from build123d import *

# Parameters (mm, degrees)
ESBO_O1_W                          = 90
ESBO_O1_H                          = 93
RESSALTO_EXTRUS_O1_DEPTH           = 12.7
ESBO_O3_R                          = 32.51
CORTE_EXTRUS_O2_DEPTH              = 66.943460631
CORTE_EXTRUS_O4_REACH              = 67.943
ESBO_O5_W                          = 27.5
ESBO_O5_H                          = 13
CORTE_EXTRUS_O5_REACH              = 67.943
ESBO_O6_W                          = 7
ESBO_O6_H                          = 26.329700269
CORTE_EXTRUS_O6_REACH              = 80.929
ESBO_O7_R                          = 2.5
CORTE_EXTRUS_O7_REACH              = 80.929
CORTE_EXTRUS_O8_DEPTH              = 66.943460631
TALADRO_DE_MARGEN_PARA_00001_D     = 5
TALADRO_DE_MARGEN_PARA_00001_DEPTH = 20
TALADRO_DE_MARGEN_PARA_00001_TIP   = 1.502151548


with BuildPart() as part:
    # Esboço1 → Ressalto-extrusão1 (new body)
    with BuildSketch(Plane(origin=(0, 0, 0), x_dir=(1, 0, 0), z_dir=(0, 1, 0))):
        Rectangle(ESBO_O1_W, ESBO_O1_H)
    extrude(amount=RESSALTO_EXTRUS_O1_DEPTH)

    # Esboço3 → Corte-extrusão2 (cut, through all)
    with BuildSketch(Plane(origin=(0, 12.7, 0), x_dir=(1, 0, 0), z_dir=(0, 1, 0))):
        with Locations(Location((0, 3.5, 0), (0, 0, 270))):
            Circle(ESBO_O3_R)
    extrude(amount=-CORTE_EXTRUS_O2_DEPTH, mode=Mode.SUBTRACT)

    # Esboço5 → Corte-extrusão4 (cut, up to next)
    with BuildSketch(Plane(origin=(0, 12.7, 0), x_dir=(1, 0, 0), z_dir=(0, 1, 0)), mode=Mode.PRIVATE) as corte_extrus_o4_sk1:
        with Locations((31.25, -40)):
            Rectangle(ESBO_O5_W, ESBO_O5_H)
    corte_extrus_o4_tool1 = extrude(corte_extrus_o4_sk1.sketch, amount=-CORTE_EXTRUS_O4_REACH, mode=Mode.PRIVATE) & part.part
    # Esboço5 → Corte-extrusão4 (cut, up to next)
    with BuildSketch(Plane(origin=(0, 12.7, 0), x_dir=(1, 0, 0), z_dir=(0, 1, 0)), mode=Mode.PRIVATE) as corte_extrus_o4_sk2:
        with Locations((-31.25, -40)):
            Rectangle(ESBO_O5_W, ESBO_O5_H)
    corte_extrus_o4_tool2 = extrude(corte_extrus_o4_sk2.sketch, amount=-CORTE_EXTRUS_O4_REACH, mode=Mode.PRIVATE) & part.part
    add(corte_extrus_o4_tool1.solids().sort_by_distance((31.25, 12.7, 40))[0], mode=Mode.SUBTRACT)
    add(corte_extrus_o4_tool2.solids().sort_by_distance((-31.25, 12.7, 40))[0], mode=Mode.SUBTRACT)

    # Esboço6 → Corte-extrusão5 (cut, up to next)
    with BuildSketch(Plane(origin=(0, 12.7, 0), x_dir=(1, 0, 0), z_dir=(0, 1, 0)), mode=Mode.PRIVATE) as corte_extrus_o5_sk1:
        with Locations((0, -33.335149866)):
            Rectangle(ESBO_O6_W, ESBO_O6_H)
    corte_extrus_o5_tool1 = extrude(corte_extrus_o5_sk1.sketch, amount=-CORTE_EXTRUS_O5_REACH, mode=Mode.PRIVATE) & part.part
    add(corte_extrus_o5_tool1.solids().sort_by_distance((0, 12.7, 33.33515))[0], mode=Mode.SUBTRACT)

    # Corte-extrusão6: up to this face of the body (flat: up to its plane)
    corte_extrus_o6_end = Plane(part.part.faces().sort_by_distance((17.5, 6.35, 40))[0])
    # Esboço7 → Corte-extrusão6 (cut, up to the picked face)
    with BuildSketch(Plane.ZY.offset(17.5), mode=Mode.PRIVATE) as corte_extrus_o6_sk1:
        with Locations((41.5, 6.35)):
            Circle(ESBO_O7_R)
    corte_extrus_o6_tool1 = split(extrude(corte_extrus_o6_sk1.sketch, amount=-CORTE_EXTRUS_O6_REACH, mode=Mode.PRIVATE), bisect_by=corte_extrus_o6_end, keep=Keep.BOTH, mode=Mode.PRIVATE)
    add(corte_extrus_o6_tool1.solids().sort_by(Axis((-17.5, 6.35, 41.5), (1, 0, 0)))[0], mode=Mode.SUBTRACT)

    # Corte-extrusão7: up to this face of the body (flat: up to its plane)
    corte_extrus_o7_end = Plane(part.part.faces().sort_by_distance((17.5, 12.518261176, 40))[0])
    # Esboço8 → Corte-extrusão7 (cut, up to the picked face)
    with BuildSketch(Plane.ZY.offset(17.5), mode=Mode.PRIVATE) as corte_extrus_o7_sk1:
        Polygon((46.5, 12.7), (40, 12.7), (46.5, 6.35), align=None)
    corte_extrus_o7_tool1 = split(extrude(corte_extrus_o7_sk1.sketch, amount=-CORTE_EXTRUS_O7_REACH, mode=Mode.PRIVATE), bisect_by=corte_extrus_o7_end, keep=Keep.BOTH, mode=Mode.PRIVATE)
    # Esboço8 → Corte-extrusão7 (cut, up to the picked face)
    with BuildSketch(Plane.ZY.offset(17.5), mode=Mode.PRIVATE) as corte_extrus_o7_sk2:
        Polygon((46.5, 0), (46.5, 6.35), (40, 0), align=None)
    corte_extrus_o7_tool2 = split(extrude(corte_extrus_o7_sk2.sketch, amount=-CORTE_EXTRUS_O7_REACH, mode=Mode.PRIVATE), bisect_by=corte_extrus_o7_end, keep=Keep.BOTH, mode=Mode.PRIVATE)
    add(corte_extrus_o7_tool1.solids().sort_by(Axis((-17.5, 10.583333, 44.333333), (1, 0, 0)))[0], mode=Mode.SUBTRACT)
    add(corte_extrus_o7_tool2.solids().sort_by(Axis((-17.5, 2.116667, 44.333333), (1, 0, 0)))[0], mode=Mode.SUBTRACT)

    # Esboço9 → Corte-extrusão8 (cut, through all)
    with BuildSketch(Plane(origin=(0, 12.7, 0), x_dir=(-1, 0, 0), z_dir=(0, 1, 0))):
        Polygon((45, 28.5), (25.5, 28.5), (17.5, 33.5), (25.5, 33.5), (45, 33.5), align=None)
        Polygon((-45, 33.5), (-25.5, 33.5), (-17.5, 33.5), (-25.5, 28.5), (-45, 28.5), align=None)
    extrude(amount=-CORTE_EXTRUS_O8_DEPTH, mode=Mode.SUBTRACT)

    # Taladro de margen para #00001
    with Locations(Plane(origin=(0, 0, -46.5), x_dir=(-1, 0, 0), z_dir=(0, 0, -1))):
        with Locations((-40, 6.35), (-25, 6.35), (40, 6.35), (25, 6.35)):
            Hole(TALADRO_DE_MARGEN_PARA_00001_D / 2, depth=TALADRO_DE_MARGEN_PARA_00001_DEPTH)
            with Locations((0, 0, -(TALADRO_DE_MARGEN_PARA_00001_DEPTH + TALADRO_DE_MARGEN_PARA_00001_TIP / 2))):  # 118° drill point
                Cone(0, TALADRO_DE_MARGEN_PARA_00001_D / 2, TALADRO_DE_MARGEN_PARA_00001_TIP, mode=Mode.SUBTRACT)


solid = part.part
Design review of the part built by this model. Coordinates are the model's own, in mm. A direction names the side the tool comes from. Coordinates: 2 decimals unless noted, no trailing zeros. Loops run counter-clockwise (first coordinate to the right, second up) from the corner with the lowest first, then second, coordinate; pieces in that order, holes last. Notation, with made-up numbers: M 56.5,7.25 L 100.5,7.25 A12 cw 100.5,25.25 Z; hole C -26.5,-18 d7. An arc over 180 degrees is marked long. Use one line per item in the form item = value.
(1) Consider section B-B (x = 7). Write out the cut boundary in (y, z).
Return value:
outline = M 0,-46.5 L 12.7,-46.5 L 12.7,-35.25 L 0,-35.25 Z; M 0,28.25 L 12.7,28.25 L 12.7,40 L 6.35,46.5 L 0,40 Z; hole C 6.35,41.5 d5
(2) Consider section A-A (z = -3.5). Write out the cut boundary in (x, y).
Return value:
outline = M -45,0 L -32.51,0 L -32.51,12.7 L -45,12.7 Z; M 32.51,0 L 45,0 L 45,12.7 L 32.51,12.7 Z
(3) Consider section C-C (y = 11.25). Write out the cut boundary in (x, z).
Return value:
outline = M -45,-46.5 L 45,-46.5 L 45,28.5 L 25.5,28.5 L 17.5,33.5 L 17.5,41.48 L 3.5,41.48 L 3.5,28.82 A32.51 cw long -3.5,28.82 L -3.5,41.48 L -17.5,41.48 L -17.5,33.5 L -25.5,28.5 L -45,28.5 Z
(4) Draft analysis for pull direction X (two halves, no side actions). For faces 4 (the face through (-45, 6, -8)), 5 (the face through (10.402, 9.569, 43.204)), 6 (the face through (23.16, 8.04, -36.36)), 7 (the face through (-26.84, 8.04, -36.36)), state which applies: pulls with the +X half, pulls with the -X half, needs draft (parallel to the pull), parting line crosses it, or undercut.
Return value:
face_4 = pulls with the -X half
face_5 = needs draft
face_6 = undercut
face_7 = undercut
(5) Consider section D-D (z = 37). Write out the cut boundary in (x, y).
Return value:
outline = M -17.5,0 L -3.5,0 L -3.5,12.7 L -17.5,12.7 Z; M 3.5,0 L 17.5,0 L 17.5,12.7 L 3.5,12.7 Z
(6) For faces 1 (the face through (-35, 6, 28.5)), 2 (the face through (17.5, 6.4, 38.6)), 3 (the face through (-37.615, 7.101, -36.36)), list the 3-axis set-ups (+Z, -Z, +X, -X, +Y, -Y) from which the entire face can be reached by the end or side of a thin tool; tool diameter is ignored.
Return value:
face_1 = +Z, -X, +Y, -Y
face_2 = +Z, +X, +Y, -Y
face_3 = -Z
(7) For line 1 along Y through (x, z) = (40, -39); line 2 along Z through (x, y) = (10.5, 5); line 3 along X through (y, z) = (6.35, -33), list the stretches that pass through material, from the lowest coordinate up. Write a range as from..to.
Return value:
line_1 = 0..3.85, 8.85..12.7
line_2 = -46.5..-34.27, 27.27..39.4, 43.6..45.12
line_3 = -45..-42.5, -37.5..-27.5, -22.5..-13.66, 13.66..22.5, 27.5..37.5, 42.5..45
(8) Clearance check with flat-ended pins moving along their axes: P1, Ø6.5, axis at y = 6.35, z = 41.5, coming from the -X side; P2, Ø1.5, axis at x = -34.5, y = 2.5, coming from the +Z side; P3, Ø4.5, axis at x = -25, y = 6.35, coming from the +Z side; P4, Ø4.5, axis at y = 6.35, z = 41.5, coming from the +X side. State where each tip first meets the part, or that it passes through.
Return value:
P1 = -17.5
P2 = 28.5
P3 = 30.22
P4 = through
